```python
from build123d import *

# Parameters (mm, degrees)
CROQUIS1_R              = 7.5
SALIENTE_EXTRUIR1_DEPTH = 2
CROQUIS2_R              = 4
SALIENTE_EXTRUIR2_DEPTH = 1
CROQUIS3_R              = 1.98
CROQUIS3_R_2            = 1.18
HEMBRA_DEPTH            = 5
REDONDEO1_R             = 0.8


with BuildPart() as part:
    # Croquis1 → Saliente-Extruir1 (new body)
    with BuildSketch(Plane(origin=(0, 0, 0), x_dir=(1, 0, 0), z_dir=(0, 1, 0))):
        with Locations(Location((0, 0, 0), (0, 0, 270))):
            Circle(CROQUIS1_R)
    extrude(amount=SALIENTE_EXTRUIR1_DEPTH)

    # Croquis2 → Saliente-Extruir2 (add)
    with BuildSketch(Plane(origin=(0, 2, 0), x_dir=(1, 0, 0), z_dir=(0, 1, 0))):
        with Locations(Location((0, 0, 0), (0, 0, 270))):
            Circle(CROQUIS2_R)
    extrude(amount=SALIENTE_EXTRUIR2_DEPTH)

    # Croquis3 → Hembra (add)
    with BuildSketch(Plane(origin=(0, 3, 0), x_dir=(1, 0, 0), z_dir=(0, 1, 0))):
        with Locations(Location((0, 0, 0), (0, 0, 270))):
            Circle(CROQUIS3_R)
        with Locations(Location((0, 0, 0), (0, 0, 270))):
            Circle(CROQUIS3_R_2, mode=Mode.SUBTRACT)
    extrude(amount=HEMBRA_DEPTH)

    # Croquis4 → Cortar-Revolución1 (revolve, cut)
    with BuildSketch(Plane.XY, mode=Mode.PRIVATE) as cortar_revoluci_n1_sk:
        with BuildLine():
            Line((0, 1), (0, 0))
            Line((0, 0), (7.5, 0))
            ThreePointArc((7.5, 0), (5.304886114, 0.746987514), (3, 1))
            Line((3, 1), (0, 1))
        make_face()
    revolve(cortar_revoluci_n1_sk.sketch.rotate(Axis((0, 6.93, 0), (0, -1, 0)), 90), axis=Axis((0, 6.93, 0), (0, -1, 0)), mode=Mode.SUBTRACT)

    # Redondeo1
    redondeo1_edges = [part.edges().sort_by_distance(p)[0] for p in [
        (0, 0, -7.5),
        (0, 2, -7.5),
    ]]
    fillet(redondeo1_edges, radius=REDONDEO1_R)


solid = part.part
```
Can you work these out from the model? Positions are in its coordinate system, mm. A direction names the side the tool comes from. Coordinates: 2 decimals unless noted, no trailing zeros. Loops run counter-clockwise (first coordinate to the right, second up) from the corner with the lowest first, then second, coordinate; pieces in that order, holes last. Notation, with made-up numbers: M 75.25,73 L 84.25,73 A16 cw 84.25,90 Z; hole C -37,83 d9. An arc over 180 degrees is marked long. Put each result on its own line as item: value. Start each with the question number.
(1) I need wall thicknesses on probe 1 along X at (y, z) = (5.1, 0); probe 2 along Z at (x, y) = (0.5, 3.25); probe 3 along Y at (x, z) = (2.25, -1.25). Which ranges of each line are inside material? Lowest first, please.
(2) Imagine slicing it at B-B on y = 2.75. List the corners of the cut face in (x, z) for me, and give its area (3 significant figures).
(3) Will these pins go through, and if not, where does the flat tip stop? pin 1 Ø3 at (x, z) = (0, 0) entering from -Y; pin 2 Ø4 at (x, z) = (4, -2.5) entering from +Y; pin 3 Ø4 at (x, y) = (-4.5, 6) entering from -Z.
(4) Which directions (+Z, -Z, +X, -X, +Y, -Y) give clear straight access to the entire face, cutting with the end or side of a thin tool? Please do faces 1 (the face through (-1, 8, 1)), 2 (the face through (-1, 3, -2)).
(5) Imagine slicing it at A-A on y = 5. List the corners of the cut face in (x, z) for me.
(6) We'd pull the mould along Z, two halves only. Please class faces 3 (the face through (0, 1, 0)), 4 (the face through (-3, 2, 3)), 5 (the face through (-1.933, 5.465, -0.429)): +Z half, -Z half, draft (parallel to the pull), parting line (faces both ways), or undercut.
Worked answers:
1. probe 1: x = -1.98 to -1.18, 1.18 to 1.98
1. probe 2: z = -1.92 to -1.07, 1.07 to 1.92
1. probe 3: y = 1 to 3
2. outline: C 0,0 d8
2. area: 50.3 mm2
3. pin 1: stops at y = 1
3. pin 2: stops at y = 3
3. pin 3: passes through
4. face 1: +Z, -Z, +X, -X, +Y
4. face 2: +Y
5. outline: C 0,0 d3.96; hole C 0,0 d2.36
6. face 3: undercut
6. face 4: draft
6. face 5: parting line
